Geometry: final body of the model. Coordinates: model frame, mm. A direction names the side the tool comes from. Give positions to 0.01 mm unless a question says otherwise; leave off trailing zeros. Loops run counter-clockwise (first coordinate to the right, second up) from the corner with the lowest first, then second, coordinate; pieces in that order, holes last. Notation, with made-up numbers: M -1.5,70.5 L 33.5,70.5 A21 cw 33.5,85.5 Z; hole C 61.5,77.25 d9. An arc over 180 degrees is marked long. Put each result on its own line as item: value.
```python
from build123d import *

# Parameters (mm, degrees)
F0_W      = 30
F0_H      = 6
F1_DEPTH  = 4
F2_W      = 6
F2_H      = 6
F3_DEPTH  = 3
F4_R      = 1.55
F5_DEPTH  = 4
F7_DEPTH  = 3
F8_W      = 28
F8_H      = 28
F9_DEPTH  = 0.5
F11_R     = 1.49999
F12_R     = 10
F13_R     = 0.4
F10_W     = 4
F10_H     = 12
F14_DEPTH = 2.5


# Not quite as in the source:
# - a fillet or chamfer is up to 0.001 mm smaller than in the source, because OpenCascade refuses the exact size


with BuildPart() as f1:
    # F0 (on Top) → F1 (new body)
    with BuildSketch(Plane.XY):
        Rectangle(F0_W, F0_H)
    extrude(amount=F1_DEPTH)

    # F2 (on face) → F3 (join)
    with BuildSketch(Plane(origin=(0, 0, 0), x_dir=(1, 0, 0), z_dir=(0, 0, -1))):
        Rectangle(F2_W, F2_H)
    extrude(amount=F3_DEPTH)

    # F4 (on face) → F5 (cut, through all)
    with BuildSketch(Plane.XY.offset(4)):
        with Locations((-8.25, 0)):
            Circle(F4_R)
        with Locations((8.25, 0)):
            Circle(F4_R)
    extrude(amount=-F5_DEPTH, mode=Mode.SUBTRACT)

    # F6 (on Front) → F7 (join, through all)
    with BuildSketch(Plane.XZ):
        with BuildLine():
            Line((-15, 0), (-15, 4))
            Line((-15, 4), (-51, 4))
            ThreePointArc((-51, 4), (-67.9705627485, -3.0294372515), (-75, -20))
            Line((-75, -20), (-95, -20))
            Line((-95, -20), (-95, -60))
            Line((-95, -60), (-55, -60))
            Line((-55, -60), (-55, -20))
            ThreePointArc((-55, -20), (-49.1421356237, -5.8578643763), (-35, 0))
            Line((-35, 0), (-15, 0))
        make_face()
    extrude(amount=-F7_DEPTH)

    # F8 (on face) → F9 (cut)
    with BuildSketch(Plane.XZ):
        with Locations((-75, -40)):
            Rectangle(F8_W, F8_H)
    extrude(amount=-F9_DEPTH, mode=Mode.SUBTRACT)

    # F11 (radius 1.5 in the source; OpenCascade refuses exactly that, so slightly less here)
    f11_edges = [f1.edges().sort_by_distance(p)[0] for p in [
        (-15, 0, 2),
        (-15, -3, 2),
        (15, -3, 2),
    ]]
    fillet(f11_edges, radius=F11_R)

    # F12
    f12_edges = [f1.edges().sort_by_distance(p)[0] for p in [
        (-55, 1.5, -60),
        (-95, 1.5, -60),
        (-95, 1.5, -20),
        (-75, 1.5, -20),
    ]]
    fillet(f12_edges, radius=F12_R)

    # F13
    f13_edges = [f1.edges().sort_by_distance(p)[0] for p in [
        (3, -3, -1.5),
        (3, 3, -1.5),
        (-3, 3, -1.5),
        (-3, -3, -1.5),
    ]]
    fillet(f13_edges, radius=F13_R)

    # F10 (on face) → F14 (cut, through all)
    with BuildSketch(Plane.XZ.offset(-0.5)):
        Polygon((-81, -34), (-89, -34), (-89, -38), (-85, -38), (-85, -42), (-89, -42), (-89, -46), (-81, -46), align=None)
        with Locations((-75, -40)):
            Rectangle(F10_W, F10_H)
        Polygon((-61, -46), (-61, -34), (-69, -34), (-69, -38), (-65, -38), (-65, -46), align=None)
    extrude(amount=-F14_DEPTH, mode=Mode.SUBTRACT)


solid = f1.part
```
Item 1: Section D-D on x = -47. Output: boundary loops of the cut face in (y, z).
Output values:
outline: M 0,-4 L 3,-4 L 3,4 L 0,4 Z
Item 2: Section B-B on z = -36. Output: boundary loops of the cut face in (x, y), then the cut area to 3 significant figures.
Output values:
outline: M -95,0 L -89,0 L -89,3 L -95,3 Z; M -81,0.5 L -77,0.5 L -77,3 L -81,3 Z; M -73,0.5 L -69,0.5 L -69,3 L -73,3 Z; M -61,0 L -55,0 L -55,3 L -61,3 Z
area: 56.0 mm²
Item 3: Mould query, pull axis X, two halves, no side actions, for faces 1 (the flat face through (-65, 0, -23)), 2 (the flat face through (3, 0, -1)), 3 (the cylindrical face through (-6.772, 0.466, 2.028)). Classes: pulls with the +X half, pulls with the -X half, needs draft (parallel to the pull), parting line crosses it, or undercut.
Output values:
face 1: needs draft
face 2: pulls with the +X half
face 3: undercut
Item 4: Line query: probe 1 along Y at (x, z) = (-8.25, 1.45); probe 2 along X at (y, z) = (0.3, -33); probe 3 along Z at (x, y) = (-11.5, 2.1). Output: solid intervals per line, ascending. Write a range as [from, to].
Output values:
probe 1: [-3, -1.55], [1.55, 3]
probe 2: [-95, -89], [-61, -55]
probe 3: [0, 4]
Item 5: Section C-C on x = 8. Output: boundary loops of the cut face in (y, z).
Output values:
outline: M -3,0 L -1.53,0 L -1.53,4 L -3,4 Z; M 1.53,0 L 3,0 L 3,4 L 1.53,4 Z
Item 6: Pin query (flat end, axial travel): pin 1 Ø12 at (x, z) = (-79.5, -41) entering from -Y; pin 2 Ø1.2 at (x, y) = (-87, 1.5) entering from +Z; pin 3 Ø2.5 at (y, z) = (0, -1) entering from -X. Return the tip coordinate at first contact, or that it passes through.
Output values:
pin 1: y = 0.5
pin 2: z = -20.1
pin 3: x = -67.15
Item 7: Section A-A on x = -8.25. Output: boundary loops of the cut face in (y, z), then the cut area to 3 significant figures.
Output values:
outline: M -3,0 L -1.55,0 L -1.55,4 L -3,4 Z; M 1.55,0 L 3,0 L 3,4 L 1.55,4 Z
area: 11.6 mm²
Item 8: Set-up query: faces 4 (the flat face through (-65, 2, -42)), 5 (the flat face through (-61, 1, -40)), 6 (the cylindrical face through (9.728, 0.466, 2.028)). Return all of +Z, -Z, +X, -X, +Y, -Y with unobstructed straight access to the full face (end or side cutting, diameter ignored); none if empty.
Output values:
face 4: +Y, -Y
face 5: -Y
face 6: +Z, -Z
